Model file for the job. Use its own axes, mm. A direction names the side the tool comes from. Round coordinates to 2 decimals unless told otherwise and drop trailing zeros. Order: outer loops, then holes, each group sorted by start corner. A loop starts at its lowest first (then second) coordinate and runs counter-clockwise, first axis right, second up. Notation, with made-up numbers: (-23, 42) - (15, 42) arc R25 cw to (15, 71) - close; hole circle Ø6 at (23, -24). An arc over 180 degrees is marked (long way). Answer as CSV lines item,"result". Start each with the question number.
1. Band-saw the part on A-A on x = 0. List the corners of the cut face in (y, z) (3 decimals), then the cut area to 3 significant figures.
2. Pull direction Z, two halves, no side cores. Call faces 4 (the face through (1, 8.255, -2)), 5 (the face through (1, 0, -8.255)), 6 (the face through (-38.22, 3.02, 0.4)): released by +Z, released by -Z, zero draft, split by the parting line, or undercut.
3. Wall check: line 1 along X through (y, z) = (3.75, 0); line 2 along Y through (x, z) = (35, 0) (3 decimals); line 3 along X through (y, z) = (-1.75, 0). Give the ranges that are in metal, low to high. Write a range as [from, to].
4. Pin check, flat tips, straight feed: pin 1 Ø5.5 at (y, z) = (0, 0) entering from +X; pin 2 Ø1.8 at (y, z) = (1.5, 0) entering from -X. Stop position of each tip, or through.
5. Band-saw the part on B-B on y = 0. List the corners of the cut face in (x, z) (3 decimals).
6. 3-axis set-ups, long thin cutter, end or side, ignore diameter. For faces 1 (the face through (46.99, 0, -4)), 2 (the face through (29.21, 0, 0)), 3 (the face through (-29.21, 0, 0)): which of +Z, -Z, +X, -X, +Y, -Y reach the whole face in a straight line?
```python
from build123d import *

# Parameters (mm, degrees)
SKETCH1_W           = 16.51
SKETCH1_H           = 16.51
BOSS_EXTRUDE1_DEPTH = 46.99
SKETCH2_R           = 3.048
CUT_EXTRUDE1_DEPTH  = 17.78
CUT_EXTRUDE2_START  = 8.255
SKETCH3_R           = 1.27
CUT_EXTRUDE2_DEPTH  = 17.51


with BuildPart() as part:
    # Sketch1 → Boss-Extrude1 (new body, symmetric)
    with BuildSketch(Plane(origin=(0, 0, 0), x_dir=(0, 0, -1), z_dir=(1, 0, 0))):
        Rectangle(SKETCH1_W, SKETCH1_H)
    extrude(amount=BOSS_EXTRUDE1_DEPTH, both=True)

    # Sketch2 → Cut-Extrude1 (cut)
    with BuildSketch(Plane(origin=(46.99, 0, 0), x_dir=(0, 0, -1), z_dir=(1, 0, 0))):
        Circle(SKETCH2_R)
    cut_extrude1 = extrude(amount=-CUT_EXTRUDE1_DEPTH, mode=Mode.SUBTRACT)

    # Mirror1: Cut-Extrude1 across plane
    add(cut_extrude1.mirror(Plane(origin=(0, 0, 0), x_dir=(0, 0, 1), z_dir=(1, 0, 0))), mode=Mode.SUBTRACT)

    # Sketch3 → Cut-Extrude2 (cut, through all)
    with BuildSketch(Plane(origin=(0, 0, 0), x_dir=(1, 0, 0), z_dir=(0, 1, 0)).offset(CUT_EXTRUDE2_START)):
        Circle(SKETCH3_R)
    extrude(amount=-CUT_EXTRUDE2_DEPTH, mode=Mode.SUBTRACT)


solid = part.part
```
Reply:
1,outline,"(-8.255, -8.255) - (8.255, -8.255) - (8.255, -1.27) - (-8.255, -1.27) - close; (-8.255, 1.27) - (8.255, 1.27) - (8.255, 8.255) - (-8.255, 8.255) - close"
1,area,"231 mm2"
2,face 4,"zero draft"
2,face 5,"released by -Z"
2,face 6,"undercut"
3,line 1,"x = [-46.99, -1.27], [1.27, 46.99]"
3,line 2,"y = [-8.255, -3.048], [3.048, 8.255]"
3,line 3,"x = [-29.21, -1.27], [1.27, 29.21]"
4,pin 1,"stops at x = 29.21"
4,pin 2,"stops at x = -29.21"
5,outline,"(-46.99, -8.255) - (46.99, -8.255) - (46.99, -3.048) - (29.21, -3.048) - (29.21, 3.048) - (46.99, 3.048) - (46.99, 8.255) - (-46.99, 8.255) - (-46.99, 3.048) - (-29.21, 3.048) - (-29.21, -3.048) - (-46.99, -3.048) - close; hole circle Ø2.54 at (0, 0)"
6,face 1,"+Z, -Z, +X, +Y, -Y"
6,face 2,"+X"
6,face 3,"-X"
